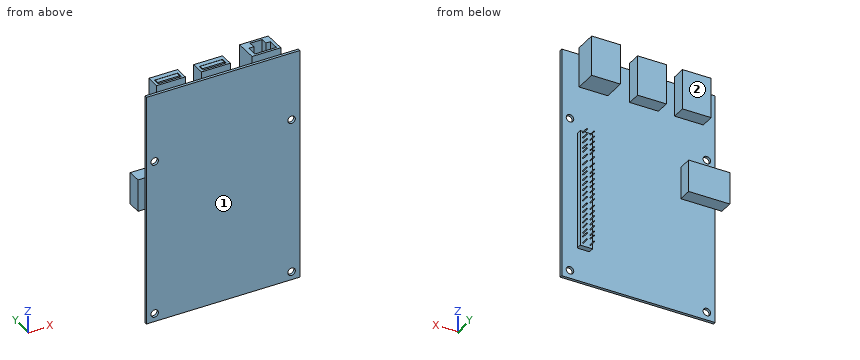
```python
from build123d import *

# Parameters (mm, degrees)
SKETCH1_W           = 56
SKETCH1_H           = 85
BOSS_EXTRUDE2_DEPTH = 1
SKETCH2_R           = 1.375
CUT_EXTRUDE1_DEPTH  = 2
SKETCH3_W           = 10.5
SKETCH3_H           = 14.7412865
BOSS_EXTRUDE3_DEPTH = 5
SKETCH5_W           = 10.5
SKETCH5_H           = 14.7412865
BOSS_EXTRUDE4_DEPTH = 3
CUT_EXTRUDE3_DEPTH  = 5
SKETCH7_W           = 15.02443759
SKETCH7_H           = 11.765446253
BOSS_EXTRUDE5_DEPTH = 5
SKETCH8_W           = 4.473595772
SKETCH8_H           = 42.973632112
BOSS_EXTRUDE6_DEPTH = 2
SKETCH9_R           = 0.150692164
SKETCH9_R_2         = 0.177318989
BOSS_EXTRUDE7_DEPTH = 2.5
SKETCH10_W          = 8.5
SKETCH10_H          = 2.441134092
SKETCH10_W_2        = 8
SKETCH10_H_2        = 1.591134092
CUT_EXTRUDE4_DEPTH  = 10


with BuildPart() as part:
    # Sketch1 → Boss-Extrude2 (new body)
    with BuildSketch(Plane(origin=(0, 0, 0), x_dir=(1, 0, 0), z_dir=(0, 1, 0))):
        Rectangle(SKETCH1_W, SKETCH1_H)
    extrude(amount=BOSS_EXTRUDE2_DEPTH)

    # Sketch2 → Cut-Extrude1 (cut)
    with BuildSketch(Plane(origin=(0, 1, 0), x_dir=(1, 0, 0), z_dir=(0, 1, 0))):
        with Locations(Location((-25, 39.5, 0), (0, 0, 270))):
            Circle(SKETCH2_R)
        with Locations(Location((-25, -17.5, 0), (0, 0, 270))):
            Circle(SKETCH2_R)
        with Locations(Location((25, -17.5, 0), (0, 0, 270))):
            Circle(SKETCH2_R)
        with Locations(Location((25, 39.5, 0), (0, 0, 270))):
            Circle(SKETCH2_R)
    extrude(amount=-CUT_EXTRUDE1_DEPTH, mode=Mode.SUBTRACT)

    # Sketch3 → Boss-Extrude3 (add)
    with BuildSketch(Plane(origin=(0, 1, 0), x_dir=(1, 0, 0), z_dir=(0, 1, 0))):
        with Locations((-18.452622363, -37.62935675)):
            Rectangle(SKETCH3_W, SKETCH3_H)
        with Locations((-2.068345025, -37.62935675)):
            Rectangle(SKETCH3_W, SKETCH3_H)
        with Locations((16.410163251, -37.62935675)):
            Rectangle(SKETCH3_W, SKETCH3_H)
    extrude(amount=BOSS_EXTRUDE3_DEPTH)

    # Sketch5 → Boss-Extrude4 (add)
    with BuildSketch(Plane(origin=(0, 6, 0), x_dir=(1, 0, 0), z_dir=(0, 1, 0))):
        with Locations((16.410163251, -37.62935675)):
            Rectangle(SKETCH5_W, SKETCH5_H)
    extrude(amount=BOSS_EXTRUDE4_DEPTH)

    # Sketch6 → Cut-Extrude3 (cut)
    with BuildSketch(Plane.XY.offset(45)):
        Polygon((18.904475678, 5.77941685), (20.539810944, 5.77941685), (20.539810944, 1.854612211), (12.690201666, 1.854612211), (12.690201666, 5.77941685), (14.521777165, 5.77941685), (14.521777165, 8.134299634), (18.904475678, 8.134299634), align=None)
    extrude(amount=-CUT_EXTRUDE3_DEPTH, mode=Mode.SUBTRACT)

    # Sketch7 → Boss-Extrude5 (add)
    with BuildSketch(Plane(origin=(0, 1, 0), x_dir=(1, 0, 0), z_dir=(0, 1, 0))):
        with Locations((-22.987781205, -5.882723127)):
            Rectangle(SKETCH7_W, SKETCH7_H)
    extrude(amount=BOSS_EXTRUDE5_DEPTH)

    # Sketch8 → Boss-Extrude6 (add)
    with BuildSketch(Plane(origin=(0, 1, 0), x_dir=(1, 0, 0), z_dir=(0, 1, 0))):
        with Locations((20.101252547, 8.8708907)):
            Rectangle(SKETCH8_W, SKETCH8_H)
    extrude(amount=BOSS_EXTRUDE6_DEPTH)

    # Sketch9 → Boss-Extrude7 (add)
    with BuildSketch(Plane(origin=(0, 3, 0), x_dir=(1, 0, 0), z_dir=(0, 1, 0))):
        with Locations(Location((18.731333841, 29.224207716, 0), (0, 0, 270))):
            Circle(SKETCH9_R)
        with Locations(Location((21.39111867, 29.224207716, 0), (0, 0, 270))):
            Circle(SKETCH9_R_2)
        with Locations(Location((21.39111867, 26.863865293, 0), (0, 0, 90))):
            Circle(SKETCH9_R_2)
        with Locations(Location((18.731333841, 26.863865293, 0), (0, 0, 90))):
            Circle(SKETCH9_R)
        with Locations(Location((21.39111867, 19.643989812, 0), (0, 0, 90))):
            Circle(SKETCH9_R_2)
        with Locations(Location((18.731333841, 19.643989812, 0), (0, 0, 90))):
            Circle(SKETCH9_R)
        with Locations(Location((18.731333841, 25.466925578, 0), (0, 0, 270))):
            Circle(SKETCH9_R)
        with Locations(Location((21.39111867, 25.466925578, 0), (0, 0, 270))):
            Circle(SKETCH9_R_2)
        with Locations(Location((21.39111867, 23.40127195, 0), (0, 0, 90))):
            Circle(SKETCH9_R_2)
        with Locations(Location((18.731333841, 23.40127195, 0), (0, 0, 90))):
            Circle(SKETCH9_R)
        with Locations(Location((21.39111867, 21.562299043, 0), (0, 0, 270))):
            Circle(SKETCH9_R_2)
        with Locations(Location((18.731333841, 21.562299043, 0), (0, 0, 270))):
            Circle(SKETCH9_R)
        with Locations(Location((21.39111867, 17.692041416, 0), (0, 0, 270))):
            Circle(SKETCH9_R_2)
        with Locations(Location((18.731333841, 17.692041416, 0), (0, 0, 270))):
            Circle(SKETCH9_R)
        with Locations(Location((21.39111867, 15.773732186, 0), (0, 0, 90))):
            Circle(SKETCH9_R_2)
        with Locations(Location((18.731333841, 15.773732186, 0), (0, 0, 90))):
            Circle(SKETCH9_R)
        with Locations(Location((18.731333841, 13.322310221, 0), (0, 0, 270))):
            Circle(SKETCH9_R)
        with Locations(Location((21.39111867, 13.322310221, 0), (0, 0, 270))):
            Circle(SKETCH9_R_2)
        with Locations(Location((18.731333841, 11.404000991, 0), (0, 0, 90))):
            Circle(SKETCH9_R)
        with Locations(Location((21.39111867, 11.404000991, 0), (0, 0, 90))):
            Circle(SKETCH9_R_2)
        with Locations(Location((18.731333841, 7.533743365, 0), (0, 0, 90))):
            Circle(SKETCH9_R)
        with Locations(Location((21.39111867, 7.533743365, 0), (0, 0, 90))):
            Circle(SKETCH9_R_2)
        with Locations(Location((18.731333841, 5.694770457, 0), (0, 0, 270))):
            Circle(SKETCH9_R)
        with Locations(Location((21.39111867, 5.694770457, 0), (0, 0, 270))):
            Circle(SKETCH9_R_2)
        with Locations(Location((21.39111867, 3.62911683, 0), (0, 0, 90))):
            Circle(SKETCH9_R_2)
        with Locations(Location((18.731333841, 3.62911683, 0), (0, 0, 90))):
            Circle(SKETCH9_R)
        with Locations(Location((18.731333841, 9.452052595, 0), (0, 0, 270))):
            Circle(SKETCH9_R)
        with Locations(Location((21.39111867, 9.452052595, 0), (0, 0, 270))):
            Circle(SKETCH9_R_2)
        with Locations(Location((18.731333841, 2.232177114, 0), (0, 0, 270))):
            Circle(SKETCH9_R)
        with Locations(Location((21.39111867, 2.232177114, 0), (0, 0, 270))):
            Circle(SKETCH9_R_2)
        with Locations(Location((21.39111867, -0.128165309, 0), (0, 0, 90))):
            Circle(SKETCH9_R_2)
        with Locations(Location((18.731333841, -0.128165309, 0), (0, 0, 90))):
            Circle(SKETCH9_R)
        with Locations(Location((21.39111867, -12.145292971, 0), (0, 0, 90))):
            Circle(SKETCH9_R_2)
        with Locations(Location((18.731333841, -12.145292971, 0), (0, 0, 90))):
            Circle(SKETCH9_R)
        with Locations(Location((18.731333841, -2.565075067, 0), (0, 0, 270))):
            Circle(SKETCH9_R)
        with Locations(Location((21.39111867, -2.565075067, 0), (0, 0, 270))):
            Circle(SKETCH9_R_2)
        with Locations(Location((21.39111867, -4.92541749, 0), (0, 0, 90))):
            Circle(SKETCH9_R_2)
        with Locations(Location((18.731333841, -4.92541749, 0), (0, 0, 90))):
            Circle(SKETCH9_R)
        with Locations(Location((18.731333841, -6.322357206, 0), (0, 0, 270))):
            Circle(SKETCH9_R)
        with Locations(Location((21.39111867, -6.322357206, 0), (0, 0, 270))):
            Circle(SKETCH9_R_2)
        with Locations(Location((21.39111867, -8.388010833, 0), (0, 0, 90))):
            Circle(SKETCH9_R_2)
        with Locations(Location((18.731333841, -8.388010833, 0), (0, 0, 90))):
            Circle(SKETCH9_R)
        with Locations(Location((21.39111867, -10.226983741, 0), (0, 0, 270))):
            Circle(SKETCH9_R_2)
        with Locations(Location((18.731333841, -10.226983741, 0), (0, 0, 270))):
            Circle(SKETCH9_R)
    extrude(amount=BOSS_EXTRUDE7_DEPTH)

    # Sketch10 → Cut-Extrude4 (cut)
    # profile 1 of 2: a face of its own
    with BuildSketch(Plane.XY.offset(45)):
        with Locations((-18.452622363, 2.970567046)):
            Rectangle(SKETCH10_W, SKETCH10_H)
        with Locations((-18.452622363, 3.295567046)):
            Rectangle(SKETCH10_W_2, SKETCH10_H_2, mode=Mode.SUBTRACT)
    # profile 2 of 2: a face of its own
    with BuildSketch(Plane.XY.offset(45)):
        with Locations((-2.068345025, 2.970567046)):
            Rectangle(SKETCH10_W, SKETCH10_H)
        with Locations((-2.068345025, 3.295567046)):
            Rectangle(SKETCH10_W_2, SKETCH10_H_2, mode=Mode.SUBTRACT)
    extrude(amount=-CUT_EXTRUDE4_DEPTH, mode=Mode.SUBTRACT)


solid = part.part
```
Build history of the part. All positions in model axes, mm. Face numbers are marked on the shaded views. A direction names the side the tool comes from. Round coordinates to 2 decimals unless told otherwise and drop trailing zeros. Write each loop counter-clockwise with the first axis right and the second up, starting at its lowest first coordinate (ties: lowest second). Pieces come first, ordered by that corner, then holes.
1) Band-saw the part on C-C, the plane x = 25. List the corners of the cut face in (y, z) (3 decimals).
2) Drill centre lines: probe 1 along X at (y, z) = (0.65, -39.5) (3 decimals); probe 2 along X at (y, z) = (2, 33); probe 3 along Y at (x, z) = (-6, -29). Where is each one in solid material? Low to high.
3) 3-axis set-ups, long thin cutter, end or side, ignore diameter. For the marked faces 1 and 2: which of +Z, -Z, +X, -X, +Y, -Y reach the whole face in a straight line?
4) Band-saw the part on B-B, the plane x = -25. List the corners of the cut face in (y, z) (3 decimals).
5) Pin check, flat tips, straight feed: pin 1 (1.5 mm diameter, centred on y = 3, z = 6, fed in from +X); pin 2 (2.5 mm diameter, centred on y = 3.5, z = 41.5, fed in from +X); pin 3 (10 mm diameter, centred on x = -20.5, z = 17, fed in from +Y); pin 4 (1.5 mm diameter, centred on y = 3.5, z = 20.5, fed in from -X). Stop position of each tip, or through.
6) Band-saw the part on A-A, the plane z = -39.5. List the corners of the cut face in (x, y) (3 decimals).
7) Band-saw the part on D-D, the plane z = 28. List the corners of the cut face in (x, y), and give its area (3 significant figures).
Ans:
1. outline: (0, -42.5) - (1, -42.5) - (1, -40.875) - (0, -40.875) - close; (0, -38.125) - (1, -38.125) - (1, 16.125) - (0, 16.125) - close; (0, 18.875) - (1, 18.875) - (1, 42.5) - (0, 42.5) - close
2. probe 1: x = -28 to -26.375, -23.625 to 23.625, 26.375 to 28
2. probe 2: x = -23.7 to -13.2, -7.32 to 3.18, 11.16 to 21.66
2. probe 3: y = 0 to 1
3. face 1: +Z, -Z, +X, -X, -Y
3. face 2: +Z, -Z, -X, +Y
4. outline: (0, -42.5) - (1, -42.5) - (1, -40.875) - (0, -40.875) - close; (0, -38.125) - (1, -38.125) - (1, 0) - (6, 0) - (6, 11.765) - (1, 11.765) - (1, 16.125) - (0, 16.125) - close; (0, 18.875) - (1, 18.875) - (1, 42.5) - (0, 42.5) - close
5. pin 1: stops at x = 22.34
5. pin 2: stops at x = 21.66
5. pin 3: stops at y = 1
5. pin 4: passes through
6. outline: (-28, 0) - (-26.375, 0) - (-26.375, 1) - (-28, 1) - close; (-23.625, 0) - (23.625, 0) - (23.625, 1) - (-23.625, 1) - close; (26.375, 0) - (28, 0) - (28, 1) - (26.375, 1) - close
7. outline: (-28, 0) - (28, 0) - (28, 1) - (-28, 1) - close
7. area: 56.0 mm2
